Geometry check sheet. Reference: the model listing, model coordinates, mm. Face numbers are marked on the shaded views. Coordinates: 2 decimals unless noted, no trailing zeros. Loops run counter-clockwise (first coordinate to the right, second up) from the corner with the lowest first, then second, coordinate; pieces in that order, holes last.
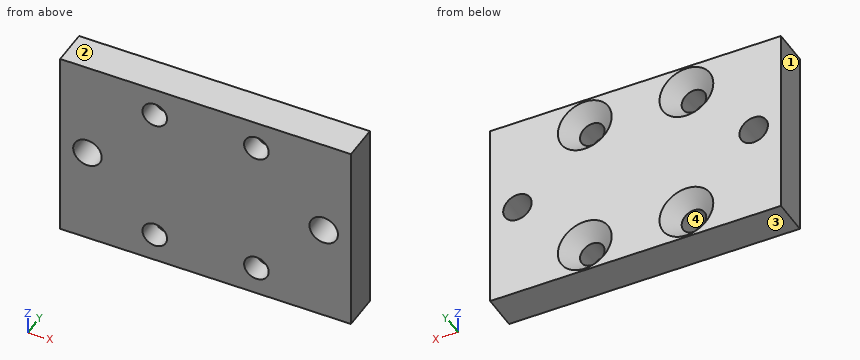
from build123d import *

# Parameters (mm, degrees)
SKETCH1_W                                       = 50.8
SKETCH1_H                                       = 33.9598
BOSS_EXTRUDE1_DEPTH                             = 6.35
SKETCH2_R                                       = 1.905
THROUGH_TO_BEARING_BLOCK_DEPTH                  = 62.434766346
SKETCH3_R                                       = 2.4892
THROUGH_TO_TNUT_DEPTH                           = 62.434766346
CSK_FOR_M4_FLAT_HEAD_MACHINE_SCREW1_D           = 4.3
CSK_FOR_M4_FLAT_HEAD_MACHINE_SCREW1_CSINK_D     = 9.4
CSK_FOR_M4_FLAT_HEAD_MACHINE_SCREW1_CSINK_ANGLE = 90


with BuildPart() as part:
    # Sketch1 → Boss-Extrude1 (new body)
    with BuildSketch(Plane(origin=(0, 0, 0), x_dir=(1, 0, 0), z_dir=(0, 1, 0))):
        with Locations((25.4, 16.9799)):
            Rectangle(SKETCH1_W, SKETCH1_H)
    extrude(amount=BOSS_EXTRUDE1_DEPTH)

    # Sketch2 → through to bearing block (cut, through all)
    with BuildSketch(Plane(origin=(0, 6.35, 0), x_dir=(1, 0, 0), z_dir=(0, 1, 0))):
        with Locations(Location((16.5227, 28.956, 0), (0, 0, 270))):
            Circle(SKETCH2_R)
        with Locations(Location((16.5227, 5.0038, 0), (0, 0, 270))):
            Circle(SKETCH2_R)
        with Locations(Location((34.2773, 28.956, 0), (0, 0, 270))):
            Circle(SKETCH2_R)
        with Locations(Location((34.2773, 5.0038, 0), (0, 0, 270))):
            Circle(SKETCH2_R)
    extrude(amount=-THROUGH_TO_BEARING_BLOCK_DEPTH, mode=Mode.SUBTRACT)

    # Sketch3 → through to tnut (cut, through all)
    with BuildSketch(Plane(origin=(0, 6.35, 0), x_dir=(1, 0, 0), z_dir=(0, 1, 0))):
        with Locations(Location((4.7625, 16.9799, 0), (0, 0, 270))):
            Circle(SKETCH3_R)
        with Locations(Location((46.0375, 16.9799, 0), (0, 0, 270))):
            Circle(SKETCH3_R)
    extrude(amount=-THROUGH_TO_TNUT_DEPTH, mode=Mode.SUBTRACT)

    # CSK for M4 Flat Head Machine Screw1 (through all)
    with Locations(Plane(origin=(0, 6.35, 0), x_dir=(1, 0, 0), z_dir=(0, 1, 0))):
        with Locations((16.5227, 28.956), (16.5227, 5.0038), (34.2773, 5.0038), (34.2773, 28.956)):
            CounterSinkHole(CSK_FOR_M4_FLAT_HEAD_MACHINE_SCREW1_D / 2, CSK_FOR_M4_FLAT_HEAD_MACHINE_SCREW1_CSINK_D / 2, counter_sink_angle=CSK_FOR_M4_FLAT_HEAD_MACHINE_SCREW1_CSINK_ANGLE)


solid = part.part
(1) Scan lines: L1, parallel to X at y = 2.25, z = -17.5; L2, parallel to Z at x = 36, y = 5.75; L3, parallel to X at y = 4.75, z = -4. Record each from-to range of solid material in increasing order.
Findings:
L1: x = 0 to 2.33, 7.2 to 43.6, 48.47 to 50.8
L2: z = -33.96 to -32.68, -25.24 to -8.72, -1.28 to 0
L3: x = 0 to 13.59, 19.46 to 31.34, 37.21 to 50.8
(2) Draft check along Z on the marked faces 1, 2, 3 and 4. Enter one of: +Z half, -Z half, draft (parallel to the pull), parting line (faces both ways), or undercut.
Findings:
face 1: draft
face 2: +Z half
face 3: -Z half
face 4: undercut
(3) Sectioned sample at A-A on y = 2.5. Record the cut outline in (x, z), and give its area (3 significant figures).
Findings:
outline: (0, -33.96) - (50.8, -33.96) - (50.8, 0) - (0, 0) - close; hole circle Ø4.98 at (4.76, -16.98); hole circle Ø4.3 at (16.52, -28.96); hole circle Ø4.3 at (16.52, -5); hole circle Ø4.3 at (34.28, -28.96); hole circle Ø4.3 at (34.28, -5); hole circle Ø4.98 at (46.04, -16.98)
area: 1,630 mm2
(4) Sectioned sample at B-B on z = -6. State how many separate pieces and enclosed holes the cut face has, and give its area (3 significant figures).
Findings:
separate pieces: 3
enclosed holes: 0
area: 260 mm2
(5) Sectioned sample at C-C on y = 5.75. Record the cut outline in (x, z).
Findings:
outline: (0, -33.96) - (50.8, -33.96) - (50.8, 0) - (0, 0) - close; hole circle Ø4.98 at (4.76, -16.98); hole circle Ø8.2 at (16.52, -28.96); hole circle Ø8.2 at (16.52, -5); hole circle Ø8.2 at (34.28, -28.96); hole circle Ø8.2 at (34.28, -5); hole circle Ø4.98 at (46.04, -16.98)
(6) Gauge pin test, flat end, axial feed: pin 1 Ø6 at (x, z) = (31, -29) entering from +Y. Record the tip position at first contact, or that the pin passes through.
Findings:
pin 1: stops at y = 6.35
